CAD build for the part. Positions are in the model's coordinates, mm. Face numbers are marked on the shaded views. A direction names the side the tool comes from. Coordinates: 2 decimals unless noted, no trailing zeros. Loops run counter-clockwise (first coordinate to the right, second up) from the corner with the lowest first, then second, coordinate; pieces in that order, holes last. Notation, with made-up numbers: (-5, -36.75) -> (38, -36.75) arc R17 cw to (38, -12.75) -> close; hole circle Ø7 at (-19, 1). An arc over 180 degrees is marked (long way). Write each question's results on one line, items separated by ' | '.
```python
from build123d import *

# Parameters (mm, degrees)
F1_DEPTH = 25.4


with BuildPart() as f1:
    # F0 (on Right) → F1 (new body)
    with BuildSketch(Plane.YZ):
        with BuildLine():
            Line((-37.447304, 15.018271), (-37.447304, 44.136662))
            Line((-37.447304, 44.136662), (-43.797303, 44.136662))
            Line((-43.797303, 44.136662), (-43.797303, 15.018271))
            ThreePointArc((-43.797303, 15.018271), (-41.937432, 10.528143), (-37.447304, 8.668271))
            Line((-37.447304, 8.668271), (-5.443305, 8.668271))
            Line((-5.443305, 8.668271), (-5.443305, 15.018271))
            Line((-5.443305, 15.018271), (-37.447304, 15.018271))
        make_face()
    extrude(amount=F1_DEPTH)


solid = f1.part
```
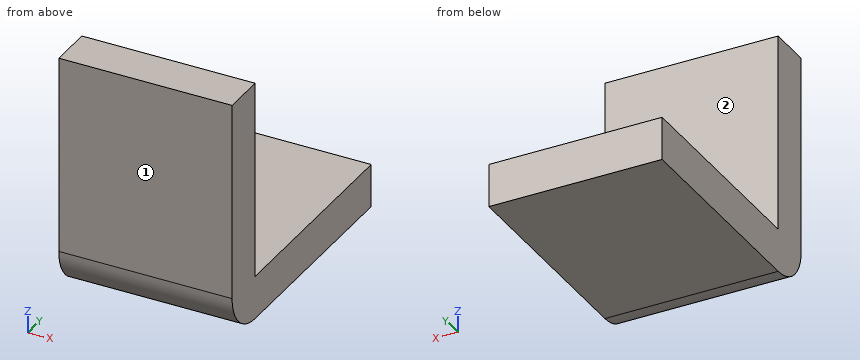
Q1. Cut at B-B on z = 33.5. Write the cut outline in (x, y).
Results are:
outline: (0, -43.8) -> (25.4, -43.8) -> (25.4, -37.45) -> (0, -37.45) -> close
Q2. Which spindle directions (+Z, -Z, +X, -X, +Y, -Y) get a long thin tool onto all of the face, cutting with end or side? Do the marked faces 1 and 2. Say none if no direction does.
Results are:
face 1: +Z, -Z, +X, -X, -Y | face 2: +Z, +X, -X, +Y
Q3. Drop flat-ended pins along their axis: pin 1 (1 mm diameter, centred on x = 6, y = -38.5, fed in from -Z); pin 2 (7.5 mm diameter, centred on x = 12, y = -23.5, fed in from +Z). Give the stop position or say it passes through.
Results are:
pin 1: z = 8.69 | pin 2: z = 15.02
Q4. Cut at C-C on y = -23. Write the cut outline in (x, z).
Results are:
outline: (0, 8.67) -> (25.4, 8.67) -> (25.4, 15.02) -> (0, 15.02) -> close
Q5. Cut at A-A on x = 13.75. Write the cut outline in (y, z), and give its area (3 significant figures).
Results are:
outline: (-43.8, 15.02) arc R6.35 ccw to (-37.45, 8.67) -> (-5.44, 8.67) -> (-5.44, 15.02) -> (-37.45, 15.02) -> (-37.45, 44.14) -> (-43.8, 44.14) -> close | area: 420 mm^2
Q6. Wall check: L1, parallel to Z at x = 20.25, y = -21; L2, parallel to Y at x = 21.25, z = 16; L3, parallel to Y at x = 19.75, z = 12. Give the ranges that are in metal, low to high. Write a range as from..to.
Results are:
L1: 8.67..15.02 | L2: -43.8..-37.45 | L3: -43.03..-5.44
